Could you check a few things on this drawing? It's one solid part, dimensions in mm from its lowest x, y, z. A direction names the side the tool comes from. Coordinates: 2 decimals unless noted, no trailing zeros. Order: outer loops, then holes, each group sorted by start corner. A loop starts at its lowest first (then second) coordinate and runs counter-clockwise, first axis right, second up. Notation, with made-up numbers: M 8,76 L 54,76 A12 cw 54,81 Z; hole C -18.5,-26 d1. An arc over 180 degrees is marked long. Answer as CSV lines item,"result". Start each with the question number.
1. I need wall thicknesses on line 1 along Y through (x, z) = (55, 2.5); line 2 along X through (y, z) = (18.5, 6.5); line 3 along Y through (x, z) = (9, 1.5). Which ranges of each line are inside material? Lowest first, please. Write a range as from..to.
2. Will these pins go through, and if not, where does the flat tip stop? pin 1 (5 mm diameter, centred on y = 6, z = 3, fed in from +X); pin 2 (5 mm diameter, centred on y = 34.5, z = 2.5, fed in from -X); pin 3 (5 mm diameter, centred on x = 53.5, z = 3, fed in from -Y).
3. If we section it at C-C (y = 20): List the corners of the cut face in (x, z) for me.
4. If we mould it in two halves opening along Y, with no side actions, what happens to the marked faces 4, 5 and 6? For each: released by +Y, released by -Y, zero draft, split by the parting line, or undercut.
5. If we section it at B-B (z = 7.75): List the corners of the cut face in (x, y) for me.
6. If we section it at A-A (x = 5): List the corners of the cut face in (y, z) for me.
7. On a 3-axis mill with a long thin cutter (end or side, diameter ignored), from which of +Z, -Z, +X, -X, +Y, -Y can I reach the whole of each face in a straight line? I mean the marked faces 1, 2 and 3. Say none if no direction works.
8. If we section it at D-D (x = 54.5): List the corners of the cut face in (y, z) for me, plus the area to 3 significant figures.
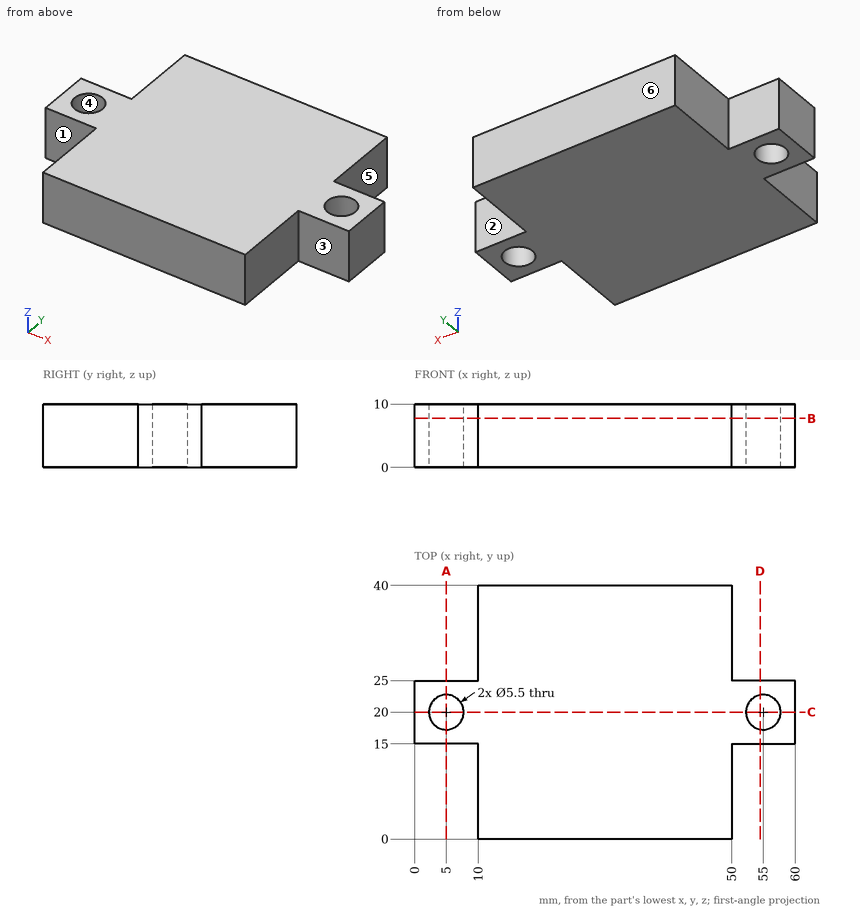
Solved:
1,line 1,"15..17.25, 22.75..25"
1,line 2,"0..2.7, 7.3..52.7, 57.3..60"
1,line 3,"15..25"
2,pin 1,"x = 50"
2,pin 2,"x = 10"
2,pin 3,"y = 15"
3,outline,"M 0,0 L 2.25,0 L 2.25,10 L 0,10 Z; M 7.75,0 L 52.25,0 L 52.25,10 L 7.75,10 Z; M 57.75,0 L 60,0 L 60,10 L 57.75,10 Z"
4,face 4,"undercut"
4,face 5,"zero draft"
4,face 6,"released by +Y"
5,outline,"M 0,15 L 10,15 L 10,0 L 50,0 L 50,15 L 60,15 L 60,25 L 50,25 L 50,40 L 10,40 L 10,25 L 0,25 Z; hole C 5,20 d5.5; hole C 55,20 d5.5"
6,outline,"M 15,0 L 17.25,0 L 17.25,10 L 15,10 Z; M 22.75,0 L 25,0 L 25,10 L 22.75,10 Z"
7,face 1,"+Z, -Z, -X, -Y"
7,face 2,"+Z, -Z, +X, +Y"
7,face 3,"+Z, -Z, +X, -Y"
8,outline,"M 15,0 L 17.3,0 L 17.3,10 L 15,10 Z; M 22.7,0 L 25,0 L 25,10 L 22.7,10 Z"
8,area,"45.9 mm²"
